```python
from build123d import *

# Parameters (mm, degrees)
SKETCH1_W           = 45.72
SKETCH1_H           = 101.6
BOSS_EXTRUDE1_DEPTH = 50.8
BOSS_EXTRUDE2_DEPTH = 50.8


with BuildPart() as part:
    # Sketch1 → Boss-Extrude1 (new body)
    with BuildSketch(Plane(origin=(0, 0, 0), x_dir=(1, 0, 0), z_dir=(0, 1, 0))):
        with Locations((22.86, 50.8)):
            Rectangle(SKETCH1_W, SKETCH1_H)
    extrude(amount=BOSS_EXTRUDE1_DEPTH)

    # Sketch4 → Boss-Extrude2 (add)
    with BuildSketch(Plane.XZ):
        with BuildLine():
            Line((0, 0), (0, 11.43))
            ThreePointArc((0, 11.43), (-5.307269755, 33.384941739), (6.985, 52.334524406))
            Line((6.985, 52.334524406), (6.985, 65.034524406))
            Line((6.985, 65.034524406), (19.685, 65.034524406))
            Line((19.685, 65.034524406), (19.685, 50.572045256))
            ThreePointArc((19.685, 50.572045256), (22.86, 6.35), (26.035, 50.572045256))
            Line((26.035, 50.572045256), (26.035, 65.034524406))
            Line((26.035, 65.034524406), (38.735, 65.034524406))
            Line((38.735, 65.034524406), (38.735, 52.334524406))
            ThreePointArc((38.735, 52.334524406), (51.027269755, 33.384941739), (45.72, 11.43))
            Line((45.72, 11.43), (45.72, 0))
            Line((45.72, 0), (0, 0))
        make_face()
    extrude(amount=-BOSS_EXTRUDE2_DEPTH)


solid = part.part
```
Design review of the part built by this model. Coordinates are the model's own, in mm. A direction names the side the tool comes from. Coordinates: 2 decimals unless noted, no trailing zeros. Order: outer loops, then holes, each group sorted by start corner. A loop starts at its lowest first (then second) coordinate and runs counter-clockwise, first axis right, second up. Notation, with made-up numbers: (-34, -4.75) - (10, -4.75) arc R16 ccw to (10, 2.25) - close; hole circle Ø8 at (22.5, 67). An arc over 180 degrees is marked (long way). Answer in a Markdown table with one row per item.
(1) Consider section D-D on x = 22.86. State the section outline as (y, z) points.
Checked values:
| item | result |
|---|---|
| outline | (0, -101.6) - (50.8, -101.6) - (50.8, 6.35) - (0, 6.35) - close |
(2) The part is to be moulded in two halves that separate along X. For faces 1 (the flat face through (23, 50.8, -36)), 2 (the flat face through (26.035, 25, 58)), 3 (the cylindrical face through (50.97, 25.04, 33.71)), say which applies: released by +X, released by -X, zero draft, split by the parting line, or undercut.
Checked values:
| item | result |
|---|---|
| face 1 | zero draft |
| face 2 | undercut |
| face 3 | released by +X |
(3) Consider section B-B on x = 31.5. State the section outline as (y, z) points, plus the area to 3 significant figures.
Checked values:
| item | result |
|---|---|
| outline | (0, -101.6) - (50.8, -101.6) - (50.8, 8.1) - (0, 8.1) - close; (0, 49.05) - (50.8, 49.05) - (50.8, 65.03) - (0, 65.03) - close |
| area | 6,380 mm^2 |
(4) Consider section C-C on z = -20. State the section outline as (x, y) points, plus the area to 3 significant figures.
Checked values:
| item | result |
|---|---|
| outline | (0, 0) - (45.72, 0) - (45.72, 50.8) - (0, 50.8) - close |
| area | 2,320 mm^2 |
(5) Clearance check with flat-ended pins moving along their axes: pin 1 (4 mm diameter, centred on y = 42.5, z = 16.5, fed in from +X); pin 2 (4.5 mm diameter, centred on y = 22, z = 60, fed in from -X) (3 decimals); pin 3 (10 mm diameter, centred on x = 11.5, z = -6.5, fed in from -Y); pin 4 (12 mm diameter, centred on y = 43, z = -65, fed in from +X). State where each tip first meets the part, or that it passes through.
Checked values:
| item | result |
|---|---|
| pin 1 | x = 49.6 |
| pin 2 | x = 6.985 |
| pin 3 | y = 0 |
| pin 4 | x = 45.72 |
(6) Wall thickness on line 1 along X through (y, z) = (46, -72); line 2 along Z through (x, y) = (22, 32); line 3 along Z through (x, y) = (32, 44.5): over which ranges is each line inside the solid? List them lowest first. Write a range as from..to.
Checked values:
| item | result |
|---|---|
| line 1 | 0..45.72 |
| line 2 | -101.6..6.37 |
| line 3 | -101.6..8.32, 48.83..65.03 |
(7) For faces 4 (the flat face through (0, 25, -46)), 5 (the flat face through (38.735, 25, 59)), 6 (the flat face through (19.685, 25, 58)), list the 3-axis set-ups (+Z, -Z, +X, -X, +Y, -Y) from which the entire face can be reached by the end or side of a thin tool; tool diameter is ignored.
Checked values:
| item | result |
|---|---|
| face 4 | -Z, -X, +Y, -Y |
| face 5 | +Z, +X, +Y, -Y |
| face 6 | +Z, +Y, -Y |
(8) Consider section A-A on y = 38. State the section outline as (x, z) points (3 decimals), plus the area to 3 significant figures.
Checked values:
| item | result |
|---|---|
| outline | (0, -101.6) - (45.72, -101.6) - (45.72, 11.43) arc R28.575 ccw to (38.735, 52.335) - (38.735, 65.035) - (26.035, 65.035) - (26.035, 50.572) arc R22.225 cw (long way) to (19.685, 50.572) - (19.685, 65.035) - (6.985, 65.035) - (6.985, 52.335) arc R28.575 ccw to (0, 11.43) - close |
| area | 6,020 mm^2 |
